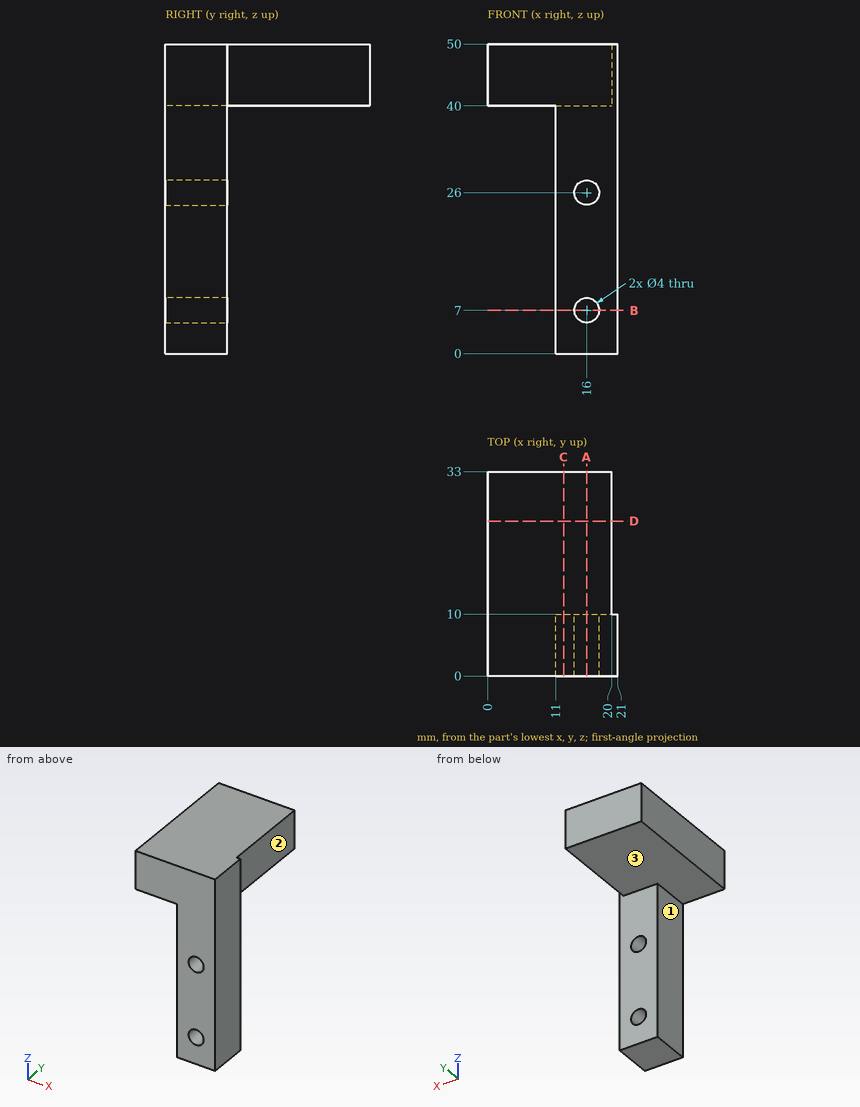
Design review of the part shown in the three views and the two pictorial views. Dimensions are in mm from the part's minimum x, y and z. A direction names the side the tool comes from. Round coordinates to 2 decimals unless told otherwise and drop trailing zeros. Write each loop counter-clockwise with the first axis right and the second up, starting at its lowest first coordinate (ties: lowest second). Pieces come first, ordered by that corner, then holes. Notation, with made-up numbers: (10, 84.5) -> (53, 84.5) arc R26 cw to (53, 112.5) -> close; hole circle Ø2 at (10.25, -15.75). An arc over 180 degrees is marked (long way). Use one line per item in the form item = value.
1) Take a section at A-A, the plane x = 16. Write out the cut boundary in (y, z), and give its area (3 significant figures).
Found:
outline = (0, 0) -> (10, 0) -> (10, 5) -> (0, 5) -> close; (0, 9) -> (10, 9) -> (10, 24) -> (0, 24) -> close; (0, 28) -> (10, 28) -> (10, 40) -> (33, 40) -> (33, 50) -> (0, 50) -> close
area = 650 mm2
2) Tool access review of the marked faces 1, 2 and 3: name each direction out of +Z, -Z, +X, -X, +Y, -Y from which nothing blocks a thin tool from reaching the whole face with its end or side.
Found:
face_1 = -Z, -X, +Y, -Y
face_2 = +Z, -Z, +X, +Y
face_3 = -Z, -X, +Y
3) To check wall thickness, follow L1, parallel to X at y = 6, z = 7; L2, parallel to Y at x = 14.5, z = 33; L3, parallel to Z at x = 4, y = 2. State the ranges of each line that lie inside material, in increasing order. Write a range as from..to.
Found:
L1 = 11..14, 18..21
L2 = 0..10
L3 = 40..50
4) Take a section at C-C, the plane x = 12.25. Write out the cut boundary in (y, z).
Found:
outline = (0, 0) -> (10, 0) -> (10, 40) -> (33, 40) -> (33, 50) -> (0, 50) -> close
5) Take a section at B-B, the plane z = 7. Write out the cut boundary in (x, y).
Found:
outline = (11, 0) -> (14, 0) -> (14, 10) -> (11, 10) -> close; (18, 0) -> (21, 0) -> (21, 10) -> (18, 10) -> close
6) Take a section at D-D, the plane y = 25. Write out the cut boundary in (x, z), and give its area (3 significant figures).
Found:
outline = (0, 40) -> (20, 40) -> (20, 50) -> (0, 50) -> close
area = 200 mm2
7) Clearance check with flat-ended pins moving along their axes: pin 1 (10 mm diameter, centred on x = 2.5, z = 31, fed in from +Y); pin 2 (10 mm diameter, centred on x = 15, z = 34.5, fed in from +Y); pin 3 (11 mm diameter, centred on y = 17.5, z = 46, fed in from +X); pin 4 (11 mm diameter, centred on y = 6.5, z = 11.5, fed in from -X). State where each tip first meets the part, or that it passes through.
Found:
pin_1 = through
pin_2 = 10
pin_3 = 20
pin_4 = 11
